Could you check a few things on this model? Use its own coordinates, in mm. Face numbers are marked on the shaded views. A direction names the side the tool comes from. Round coordinates to 2 decimals unless told otherwise and drop trailing zeros. Loops run counter-clockwise (first coordinate to the right, second up) from the corner with the lowest first, then second, coordinate; pieces in that order, holes last. Notation, with made-up numbers: (49.5, -2) -> (72.5, -2) arc R10 cw to (72.5, 3) -> close; hole circle Ø5 at (2.25, -30). An arc over 180 degrees is marked (long way). One line per item, written item: value.
Autodesk Inventor part; units mm, degrees
ref_plane "YZ Plane" through (0, 0, 0) normal (1, 0, 0) x (0, 1, 0)
ref_plane "XZ Plane" through (0, 0, 0) normal (0, 1, 0) x (-1, 0, 0)
ref_plane "XY Plane" through (0, 0, 0) normal (0, 0, 1) x (1, 0, 0)
sketch "Sketch1" plane through (0, 0, 0) normal (0, 1, 0) x (-1, 0, 0)
  line L0 (-10, 14) -> (10, 14)
  line L1 (10, 14) -> (10, -14)
  line L2 (10, -14) -> (-10, -14)
  line L3 (-10, -14) -> (-10, 14)
  line L4 (-10, 14) -> (10, -14) construction
  line L5 (10, 14) -> (-10, -14) construction
  point P0 (0, 0)
  dimension "d0" = 28
  dimension "d1" = 20
extrude "Extrusion1" add sketch "Sketch1" along normal blind 4
sketch "Sketch2" plane through (0, 4, 0) normal (0, 1, 0) x (1, 0, 0)
  line L0 (10, 14) -> (-10, 14)
  line L1 (-10, 14) -> (10, 14)
  line L2 (10, 14) -> (10, 10)
  line L3 (10, 10) -> (-10, 10)
  line L4 (-10, 10) -> (-10, 14)
  point P0 (0, 0)
  dimension "d4" = 4
extrude "Extrusion2" add sketch "Sketch2" along normal blind 24
sketch "Sketch3" plane through (0, 4, 0) normal (0, 1, 0) x (1, 0, 0)
  line L0 (-10, 10) -> (10, 10)
  line L1 (10, -14) -> (8, -14)
  line L2 (8, -14) -> (8, 10)
  line L3 (8, 10) -> (10, 10)
  line L4 (10, 10) -> (10, -14)
  line L5 (-10, -14) -> (-8, -14)
  line L6 (-8, -14) -> (-8, 10)
  line L7 (-8, 10) -> (-10, 10)
  line L8 (-10, 10) -> (-10, -14)
  point P0 (0, 0)
  dimension "d7" = 2
  dimension "d8" = 2
extrude "Extrusion3" add sketch "Sketch3" along normal blind 24
sketch "Sketch4" plane through (10, 0, 14) normal (1, 0, 0) x (0, 0, -1)
  line L0 (0, 4) -> (0, 28)
  line L1 (24, 28) -> (24, 4)
  line L2 (0, 28) -> (24, 28)
  line L3 (24, 28) -> (24, 4)
  line L4 (24, 4) -> (0, 4)
  line L5 (0, 4) -> (0, 28)
  line L6 (0, 28) -> (22, 28)
  line L7 (22, 28) -> (22, 6)
  line L8 (22, 6) -> (0, 6)
  line L9 (0, 6) -> (0, 28)
  line L10 (4, 6) -> (22, 24)
  point P0 (14, 0)
  dimension "d11" = 2
  dimension "d12" = 2
  dimension "d13" = 4
  dimension "d14" = 4
extrude "Extrusion4" cut sketch "Sketch4" against normal blind 24 contours L0 L2 L7 L10 L8
sketch "Sketch5" plane through (0, 4, 0) normal (0, 1, 0) x (1, 0, 0)
  line L0 (-8, -14) -> (8, -14)
  line L1 (0, -14) -> (0, 10)
  line L2 (-8, 10) -> (8, 10)
  line L3 (2.75, -4.75) -> (-2.75, -4.75)
  line L4 (-2.75, -4.75) -> (-2.75, 0.75)
  line L5 (-2.75, 0.75) -> (2.75, 0.75)
  line L6 (2.75, 0.75) -> (2.75, -4.75)
  line L7 (2.75, -4.75) -> (-2.75, 0.75) construction
  line L8 (-2.75, -4.75) -> (2.75, 0.75) construction
  arc A0 (2.75, 0.75) -> (-2.75, 0.75) centre (0, 0.75) ccw
  arc A1 (-2.75, -4.75) -> (2.75, -4.75) centre (0, -4.75) ccw
  point P0 (0, 0)
  point P1 (0, -2)
  dimension "d17" = 5.5
  dimension "d18" = 5.5
extrude "Extrusion5" cut sketch "Sketch5" against normal blind 24
sketch "Sketch6" plane through (-8, 4, -10) normal (0, 0, 1) x (1, 0, 0)
  line L0 (0, 24) -> (16, 24)
  line L1 (8, 24) -> (8, 0)
  line L2 (10.75, 9.25) -> (5.25, 9.25)
  line L3 (5.25, 9.25) -> (5.25, 14.75)
  line L4 (5.25, 14.75) -> (10.75, 14.75)
  line L5 (10.75, 14.75) -> (10.75, 9.25)
  line L6 (10.75, 9.25) -> (5.25, 14.75) construction
  line L7 (5.25, 9.25) -> (10.75, 14.75) construction
  arc A0 (10.75, 14.75) -> (5.25, 14.75) centre (8, 14.75) ccw
  arc A1 (5.25, 9.25) -> (10.75, 9.25) centre (8, 9.25) ccw
  line L8 (0, 0) -> (16, 0)
  point P0 (8, 12)
  dimension "d21" = 5.5
  dimension "d22" = 5.5
extrude "Extrusion6" cut sketch "Sketch6" against normal blind 24
properties part number "2020-90"
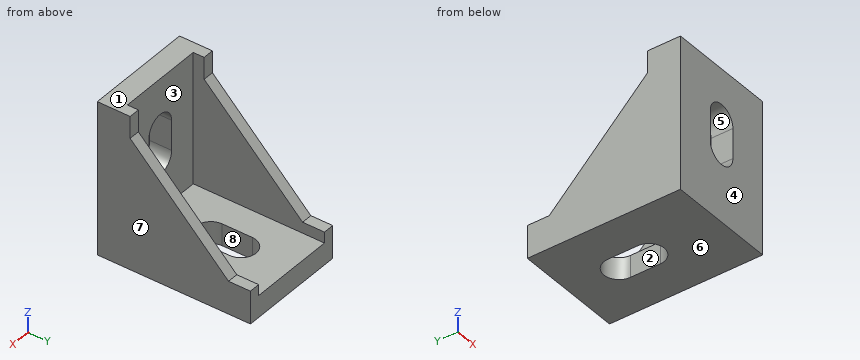
Item 1: For the marked faces 1, 2, 3, 4 and 5, which set-ups out of +Z, -Z, +X, -X, +Y, -Y let a thin tool reach every point of the face, with its end or its side?
Output:
face 1: +Z, +X, -X, +Y, -Y
face 2: +Z, -Z
face 3: +Z, +Y
face 4: +Z, -Z, +X, -X, -Y
face 5: +Y, -Y
Item 2: If we section it at A-A on z = 3.5: List the corners of the cut face in (x, y) for me.
Output:
outline: (-10, 0) -> (-2.75, 0) -> (-2.75, 4) -> (-8, 4) -> (-8, 12.5) -> (-10, 12.5) -> close; (2.75, 0) -> (10, 0) -> (10, 12.5) -> (8, 12.5) -> (8, 4) -> (2.75, 4) -> close
Item 3: If we section it at B-B on x = 0: List the corners of the cut face in (y, z) for me.
Output:
outline: (0, -14) -> (10.5, -14) -> (10.5, -10) -> (4, -10) -> (4, -3.5) -> (0, -3.5) -> close; (0, 7.5) -> (4, 7.5) -> (4, 14) -> (0, 14) -> close; (21.5, -14) -> (28, -14) -> (28, -10) -> (21.5, -10) -> close
Item 4: If we section it at D-D on z = 9.5: List the corners of the cut face in (x, y) for me, plus the area to 3 significant figures.
Output:
outline: (-10, 0) -> (10, 0) -> (10, 6.5) -> (8, 6.5) -> (8, 4) -> (-8, 4) -> (-8, 6.5) -> (-10, 6.5) -> close
area: 90.0 mm²
Item 5: If we section it at C-C on y = 2.75: List the corners of the cut face in (x, z) for me, plus the area to 3 significant figures.
Output:
outline: (-10, -14) -> (10, -14) -> (10, 14) -> (-10, 14) -> close; hole (-2.75, -0.75) arc R2.75 ccw to (2.75, -0.75) -> (2.75, 4.75) arc R2.75 ccw to (-2.75, 4.75) -> close
area: 506 mm²
Item 6: Will these pins go through, and if not, where does the flat tip stop? pin 1 Ø2 at (x, y) = (7.5, 10.5) entering from +Z; pin 2 Ø1.5 at (x, y) = (-6, 22.5) entering from +Z; pin 3 Ø3 at (x, z) = (5.5, 1) entering from -Y; pin 4 Ø1.6 at (x, y) = (-9, 25) entering from +Z.
Output:
pin 1: stops at z = 6.37
pin 2: stops at z = -10
pin 3: stops at y = 0
pin 4: stops at z = -8
Item 7: If we mould it in two halves opening along X, with no side actions, what happens to the marked faces 6, 7 and 8? For each: released by +X, released by -X, zero draft, split by the parting line, or undercut.
Output:
face 6: zero draft
face 7: released by +X
face 8: undercut
Item 8: I need wall thicknesses on line 1 (X direction, y = 13.75, z = -12); line 2 (X direction, y = 7.5, z = -3.5); line 3 (Y direction, x = 6, z = -8.25). Which ranges of each line are inside material? Lowest first, please. Write a range as from..to.
Output:
line 1: x = -10..-2.75, 2.75..10
line 2: x = -10..-8, 8..10
line 3: y = 0..4
